Verification items for the finished model (mm, model axes). Face numbers are marked on the shaded views. Coordinates: 2 decimals unless noted, no trailing zeros. Loops run counter-clockwise (first coordinate to the right, second up) from the corner with the lowest first, then second, coordinate; pieces in that order, holes last. Notation, with made-up numbers: (83.25, -32) - (107.25, -32) arc R22 cw to (107.25, 0) - close; hole circle Ø2 at (10, 42.5). An arc over 180 degrees is marked (long way). Answer as CSV lines item,"result". Start each with the question number.
1. Cross-section at A-A (y = -51.5). Enter the section's corners in (x, z).
2. Cross-section at D-D (z = -811). Enter the section's corners in (x, y).
3. Gauge pin test, flat ends, axial feed: P1, Ø6, axis at y = 130, z = -470.5, coming from the -X side; P2, Ø8, axis at y = 87.5, z = -385, coming from the +X side; P3, Ø9, axis at x = -195, z = 35, coming from the -Y side. Record the tip position at first contact, or that the pin passes through.
4. Cross-section at C-C (y = 174.5). Enter the section's corners in (x, z), plus the area to 3 significant figures.
5. Material ranges on line 1 (X direction, y = 215.5, z = 35); line 2 (Z direction, x = 195, y = -211.5); line 3 (Z direction, x = -202, y = -54.5), recorded low to high. Write a range as [from, to].
6. Cross-section at B-B (x = 79.5). Enter the section's corners in (y, z).
7. Release check for a two-part mould opening along Z. For the marked faces 1, 2 and 3 record: pulls with the +Z half, pulls with the -Z half, needs draft (parallel to the pull), parting line crosses it, or undercut.
```python
from build123d import *

# Parameters (mm, degrees)
EXTRUDE_1_DEPTH          = 70
CUT_EXTRUDE_1_DEPTH      = 1
CUT_EXTRUDE_1_DEPTH_BACK = 65
SKETCH_4_R               = 2
CUT_EXTRUDE_2_DEPTH      = 10
SKETCH_3_R               = 5
CUT_EXTRUDE_3_DEPTH      = 10
EXTRUDE_2_DEPTH          = 10
EXTRUDE_3_DEPTH          = 435


with BuildPart() as part:
    # 草图1 → 凸台-拉伸1 (new body)
    with BuildSketch(Plane.XY):
        Polygon((225, 0), (225, 217.5), (-225, 217.5), (-225, 0), (-225, -217.5), (225, -217.5), align=None)
    extrude(amount=EXTRUDE_1_DEPTH)

    # 草图2 → 切除-拉伸1 (cut, two sides)
    with BuildSketch(Plane.XY.offset(70)) as cut_extrude_1_sk:
        Polygon((0, 217.5), (-100, 217.5), (-100, 151.164004593), (-225, 151.164004593), (-225, -151.164004593), (-100, -151.164004593), (-100, -217.5), (100, -217.5), (100, -151.164004593), (225, -151.164004593), (225, 151.164004593), (100, 151.164004593), (100, 217.5), align=None)
    extrude(amount=CUT_EXTRUDE_1_DEPTH, mode=Mode.SUBTRACT)
    extrude(cut_extrude_1_sk.sketch, amount=-CUT_EXTRUDE_1_DEPTH_BACK, mode=Mode.SUBTRACT)

    # 草图4 → 切除-拉伸2 (cut)
    with BuildSketch(Plane.XY.offset(5)):
        with Locations((215, 0)):
            Circle(SKETCH_4_R)
    extrude(amount=-CUT_EXTRUDE_2_DEPTH, mode=Mode.SUBTRACT)

    # 草图3 → 切除-拉伸3 (cut)
    with BuildSketch(Plane(origin=(0, 217.5, 0), x_dir=(1, 0, 0), z_dir=(0, 1, 0))):
        with Locations((-195, -35)):
            Circle(SKETCH_3_R)
        with Locations((195, -35)):
            Circle(SKETCH_3_R)
    cut_extrude_3 = extrude(amount=-CUT_EXTRUDE_3_DEPTH, mode=Mode.SUBTRACT)

    # 镜向1: 切除-拉伸3 across plane
    add(cut_extrude_3.mirror(Plane.ZX), mode=Mode.SUBTRACT)

    # 草图6 → 凸台-拉伸2 (add)
    with BuildSketch(Plane(origin=(0, -217.5, 0), x_dir=(-1, 0, 0), z_dir=(0, -1, 0))):
        Polygon((-15.031554005, 140), (-225.473310071, 0), (-225, 0), (-195.410202062, 0), (0, 130), (195.410202062, 0), (225, 0), (225.473310071, 0), (15.031554005, 140), (255.536418081, 300), (225.473310071, 300), (0, 150), (-225.473310071, 300), (-255.536418081, 300), align=None)
    extrude_2 = extrude(amount=-EXTRUDE_2_DEPTH)

    # 镜向2: 凸台-拉伸2 across plane
    add(extrude_2.mirror(Plane.ZX))

    # 草图7 → 凸台-拉伸3 (add)
    with BuildSketch(Plane(origin=(0, 217.5, 0), x_dir=(1, 0, 0), z_dir=(0, 1, 0))):
        Polygon((-255.536418081, 300), (255.536418081, 300), (458.675595133, 0), (476.639391287, 0), (260.073177672, 319.829316172), (-237.490096329, 319.829316172), (-472.660078337, 868.671562843), (-498.536821512, 868.671562843), align=None)
    extrude(amount=-EXTRUDE_3_DEPTH)


solid = part.part
```
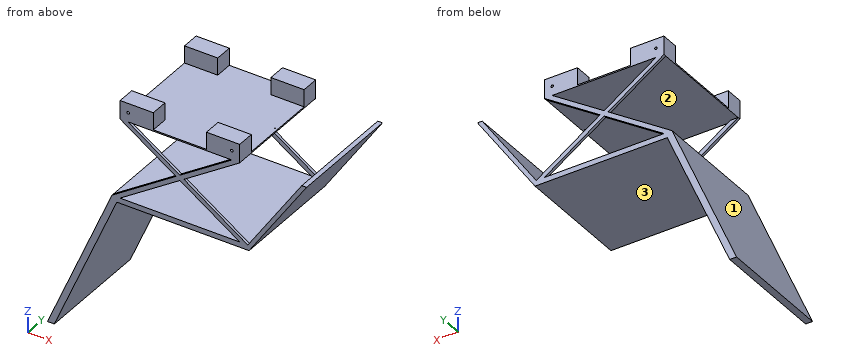
Values follow:
1,outline,"(-498.54, -868.67) - (-472.66, -868.67) - (-237.49, -319.83) - (260.07, -319.83) - (476.64, 0) - (458.68, 0) - (255.54, -300) - (-255.54, -300) - close; (-225, 0) - (225, 0) - (225, 5) - (-225, 5) - close"
2,outline,"(-473.89, -217.5) - (-447.95, -217.5) - (-447.95, 217.5) - (-473.89, 217.5) - close"
3,P1,"stops at x = -329.68"
3,P2,"stops at x = -263.7"
3,P3,"stops at y = -207.5"
4,outline,"(-498.54, -868.67) - (-472.66, -868.67) - (-237.49, -319.83) - (260.07, -319.83) - (476.64, 0) - (458.68, 0) - (255.54, -300) - (-255.54, -300) - close; (-225, 0) - (225, 0) - (225, 70) - (100, 70) - (100, 5) - (-100, 5) - (-100, 70) - (-225, 70) - close"
4,area,"48,700 mm²"
5,line 1,"x = [-225, -200], [-190, -100], [100, 190], [200, 225]"
5,line 2,"z = [-319.83, -300], [-279.73, -259.73], [-20.27, -0.27], [0, 30], [40, 70]"
5,line 3,"z = [-319.83, -300], [0, 5]"
6,outline,"(-217.5, -319.83) - (217.5, -319.83) - (217.5, -300) - (-217.5, -300) - close; (-217.5, -202.89) - (-207.5, -202.89) - (-207.5, -182.89) - (-217.5, -182.89) - close; (-217.5, -97.11) - (-207.5, -97.11) - (-207.5, -77.11) - (-217.5, -77.11) - close; (-217.5, 0) - (217.5, 0) - (217.5, 5) - (-217.5, 5) - close; (207.5, -202.89) - (217.5, -202.89) - (217.5, -182.89) - (207.5, -182.89) - close; (207.5, -97.11) - (217.5, -97.11) - (217.5, -77.11) - (207.5, -77.11) - close"
7,face 1,"pulls with the +Z half"
7,face 2,"undercut"
7,face 3,"pulls with the -Z half"
